Geometry check sheet. Reference: the model listing, model coordinates, mm. A direction names the side the tool comes from. Round coordinates to 2 decimals unless told otherwise and drop trailing zeros. Write each loop counter-clockwise with the first axis right and the second up, starting at its lowest first coordinate (ties: lowest second). Pieces come first, ordered by that corner, then holes. Notation, with made-up numbers: (-16.75, -32.5) - (39.25, -32.5) arc R11 cw to (39.25, -19.5) - close; hole circle Ø8 at (53, -35.5). An arc over 180 degrees is marked (long way). Return JSON: item names as keys, results as strings. Group by question number.
Autodesk Inventor part; units mm, degrees
ref_plane "YZ Plane" through (0, 0, 0) normal (1, 0, 0) x (0, 1, 0)
ref_plane "XZ Plane" through (0, 0, 0) normal (0, 1, 0) x (-1, 0, 0)
ref_plane "XY Plane" through (0, 0, 0) normal (0, 0, 1) x (1, 0, 0)
sketch "Sketch1" plane through (0, 0, 0) normal (0, 0, 1) x (1, 0, 0)
  line L0 (-14.75, -15.25) -> (14.75, -15.25)
  line L1 (14.75, -15.25) -> (14.75, 15.25)
  line L2 (14.75, 15.25) -> (-14.75, 15.25)
  line L3 (-14.75, 15.25) -> (-14.75, -15.25)
  line L4 (-14.75, -15.25) -> (14.75, 15.25) construction
  line L5 (14.75, -15.25) -> (-14.75, 15.25) construction
  point P0 (0, 0)
  dimension "WIDTH" = 29.5
  dimension "LENGTH" = 30.5
extrude "Extrusion1" add sketch "Sketch1" along normal blind 4.55
sketch "Sketch4" plane through (0, 0, 4.55) normal (0, 0, 1) x (1, 0, 0)
  line L0 (-14.75, 24.75) -> (14.75, 24.75)
  line L1 (14.75, 24.75) -> (14.75, -24.75)
  line L2 (14.75, -24.75) -> (-14.75, -24.75)
  line L3 (-14.75, -24.75) -> (-14.75, 24.75)
  line L4 (-14.75, 24.75) -> (14.75, -24.75) construction
  line L5 (14.75, 24.75) -> (-14.75, -24.75) construction
  point P0 (0, 0)
  dimension "LENGTH_WHOLE" = 49.5
  dimension "d30" = 29.5
extrude "Extrusion2" add sketch "Sketch4" against normal blind 4.55
sketch "Sketch2" plane through (0, 0, 4.55) normal (0, 0, 1) x (1, 0, 0)
  point P0 (0, 0)
  point P1 (-11, 6)
  point P2 (11, 6)
  point P3 (-11, -6)
  point P4 (11, -6)
  dimension "d11" = 22
  dimension "d12" = 0
  dimension "d13" = 0
  dimension "d14" = 0
  dimension "d15" = 0
  dimension "d16" = 12
  dimension "d17" = 6
  dimension "d18" = 11
hole "Hole1" at (-11, 6, 4.55) at (11, 6, 4.55) at (-11, -6, 4.55) at (11, -6, 4.55) direction (0, 0, -1) diameter 2.4 end through all counterbore diameter 4.4 counterbore depth 2.1
sketch "Sketch5" plane through (0, 0, 0) normal (0, 0, -1) x (-1, 0, 0)
  point P0 (0, 0)
  point P1 (0, 20)
  point P2 (0, -20)
  dimension "d40" = 0
  dimension "d41" = 0
  dimension "d42" = 20
  dimension "d43" = 40
hole "Hole3" at (0, 20, 0) at (0, -20, 0) direction (0, 0, 1) diameter 4.5 end through all
sketch "Sketch9" plane through (0, 0, 0) normal (0, 0, -1) x (-1, 0, 0)
  circle A0 centre (11, 6) radius 1.2
  point P0 (0, 0)
  point P1 (11, -6)
  point P2 (-11, 6)
  point P3 (-11, -6)
  dimension "d79" = 0
  dimension "d80" = 0
  dimension "d81" = 0
  dimension "d82" = 12
  dimension "d83" = 0
  dimension "d84" = 22
  dimension "d85" = 0
  dimension "d86" = 0
hole "Hole6" at (-11, 6, 0) at (-11, -6, 0) at (11, 6, 0) at (11, -6, 0) direction (0, 0, 1) diameter 3.75 depth 0.5
chamfer "Chamfer3" distance 1 angle 45 4 edges at (14.75, -24.75, 2.275) (-14.75, -24.75, 2.275) (-14.75, 24.75, 2.275) (14.75, 24.75, 2.275)
equation "\"d30\" = WIDTH"
properties part number "camera_mount"
1. Tool access check on faces 1 (the face through (-11.66, 3.9, 3.49)), 2 (the face through (0, 24.75, 2)), 3 (the face through (-9.17, 5.59, 0.25)). Record the directions out of +Z, -Z, +X, -X, +Y, -Y that give a thin tool (end or side, any length) a straight path to the whole face; none if there is none.
2. Section check D-D (y = -6). Enter the section's corners in (x, z) (3 decimals).
3. Section check C-C (z = 1.8). Enter the section's corners in (x, y), and give its area (3 significant figures).
4. Section check A-A (x = 0). Enter the section's corners in (y, z).
5. Material ranges on line 1 along Y through (x, z) = (0, 1); line 2 along X through (y, z) = (-6, 0.2) (3 decimals); line 3 along Y through (x, z) = (11, 3.6), recorded low to high.
6. Depth check by flat-ended pin: pin 1 Ø1.9 at (x, y) = (11.5, -5.5) entering from -Z; pin 2 Ø2.5 at (x, y) = (-11, 6) entering from +Z; pin 3 Ø2 at (x, y) = (-11, -6) entering from -Z. Enter the tip coordinate at first touch or a pass-through.
7. Section check B-B (y = -20). Enter the section's corners in (x, z).
8. Mould release check, pull along X, two halves, no side actions. Record for faces 4 (the face through (-14.2, -24.3, 2.3)), 5 (the face through (14.3, 24.2, 2.2)), 6 (the face through (-0.676, 22.146, 2.307)): pulls with the +X half, pulls with the -X half, needs draft (parallel to the pull), parting line crosses it, or undercut.
Result sheet:
{
 "1": {"face 1": "+Z", "face 2": "+Z, -Z, +X, -X, +Y", "face 3": "-Z"},
 "2": {"outline": "(-14.75, 0) - (-12.875, 0) - (-12.875, 0.5) - (-12.2, 0.5) - (-12.2, 2.45) - (-13.2, 2.45) - (-13.2, 4.55) - (-14.75, 4.55) - close; (-9.8, 0.5) - (-9.125, 0.5) - (-9.125, 0) - (9.125, 0) - (9.125, 0.5) - (9.8, 0.5) - (9.8, 2.45) - (8.8, 2.45) - (8.8, 4.55) - (-8.8, 4.55) - (-8.8, 2.45) - (-9.8, 2.45) - close; (12.2, 0.5) - (12.875, 0.5) - (12.875, 0) - (14.75, 0) - (14.75, 4.55) - (13.2, 4.55) - (13.2, 2.45) - (12.2, 2.45) - close"},
 "3": {"outline": "(-14.75, -23.75) - (-13.75, -24.75) - (13.75, -24.75) - (14.75, -23.75) - (14.75, 23.75) - (13.75, 24.75) - (-13.75, 24.75) - (-14.75, 23.75) - close; hole circle Ø2.4 at (-11, -6); hole circle Ø2.4 at (-11, 6); hole circle Ø4.5 at (0, -20); hole circle Ø4.5 at (0, 20); hole circle Ø2.4 at (11, -6); hole circle Ø2.4 at (11, 6)", "area": "1,410 mm²"},
 "4": {"outline": "(-24.75, 0) - (-22.25, 0) - (-22.25, 4.55) - (-24.75, 4.55) - close; (-17.75, 0) - (17.75, 0) - (17.75, 4.55) - (-17.75, 4.55) - close; (22.25, 0) - (24.75, 0) - (24.75, 4.55) - (22.25, 4.55) - close"},
 "5": {"line 1": "y = -24.75 to -22.25, -17.75 to 17.75, 22.25 to 24.75", "line 2": "x = -14.75 to -12.875, -9.125 to 9.125, 12.875 to 14.75", "line 3": "y = -24.75 to -8.2, -3.8 to 3.8, 8.2 to 24.75"},
 "6": {"pin 1": "stops at z = 0.5", "pin 2": "stops at z = 2.45", "pin 3": "passes through"},
 "7": {"outline": "(-14.75, 0) - (-2.25, 0) - (-2.25, 4.55) - (-14.75, 4.55) - close; (2.25, 0) - (14.75, 0) - (14.75, 4.55) - (2.25, 4.55) - close"},
 "8": {"face 4": "pulls with the -X half", "face 5": "pulls with the +X half", "face 6": "undercut"}
}
